Geometry check sheet. Reference: the model listing, model coordinates, mm. Round coordinates to 2 decimals unless told otherwise and drop trailing zeros. Write each loop counter-clockwise with the first axis right and the second up, starting at its lowest first coordinate (ties: lowest second). Pieces come first, ordered by that corner, then holes. Notation, with made-up numbers: (57, 65.25) -> (102, 65.25) arc R22 ccw to (102, 90.25) -> close; hole circle Ø7 at (57.25, -36). An arc over 180 degrees is marked (long way). One line per question, with ' | ' between items.
```python
from build123d import *

# Parameters (mm, degrees)
SKETCH3_R           = 1
BOSS_EXTRUDE2_DEPTH = 1.5
MOVE_FACE1_BY       = 0.2
MOVE_FACE1_2_BY     = 0.2


with BuildPart() as part:
    # Sketch3 → Boss-Extrude2 (new body)
    with BuildSketch(Plane(origin=(0, 0, 0), x_dir=(1, 0, 0), z_dir=(0, 1, 0))):
        with BuildLine():
            Line((9.052045009, -11.69440211), (-2.494704275, -15.782345478))
            Line((-2.494704275, -15.782345478), (-2.714831854, -15.909670913))
            Line((-2.714831854, -15.909670913), (-5.018414472, -17.242101226))
            ThreePointArc((-5.018414472, -17.242101226), (-5.90236336, -19.640824396), (-3.706036939, -20.949024969))
            Line((-3.706036939, -20.949024969), (-1.077229318, -20.535220782))
            Line((-1.077229318, -20.535220782), (-0.82602363, -20.495678153))
            Line((-0.82602363, -20.495678153), (10.720725655, -16.407734785))
            Line((10.720725655, -16.407734785), (13.853836403, -15.298506639))
            ThreePointArc((13.853836403, -15.298506639), (14.422653253, -14.786418923), (14.462766809, -14.022103975))
            Line((14.462766809, -14.022103975), (14.300666867, -13.564238683))
            Line((14.300666867, -13.564238683), (13.487374274, -11.195126647))
            ThreePointArc((13.487374274, -11.195126647), (12.976450881, -10.619337061), (12.207817887, -10.577150797))
            Line((12.207817887, -10.577150797), (9.052045009, -11.69440211))
        make_face()
        with Locations(Location((-4.01703029, -18.973352138, 0), (0, 0, 270))):
            Circle(SKETCH3_R, mode=Mode.SUBTRACT)
        with Locations(Location((12.007385036, -13.300162157, 0), (0, 0, 270))):
            Circle(SKETCH3_R, mode=Mode.SUBTRACT)
    extrude(amount=BOSS_EXTRUDE2_DEPTH)

    # Move Face1: a curved face moved inward by 0.2
    add(Solid.thicken(part.faces().sort_by_distance((12.007385036, 0.75, 12.300162157))[0], -MOVE_FACE1_BY), mode=Mode.SUBTRACT)

    # Move Face1 2: a curved face moved inward by 0.2
    add(Solid.thicken(part.faces().sort_by_distance((-4.01703029, 0.75, 17.973352138))[0], -MOVE_FACE1_2_BY), mode=Mode.SUBTRACT)


solid = part.part
```
(1) Sectioned sample at B-B on z = 13. Record the cut outline in (x, y).
Resolved:
outline: (5.36, 0) -> (10.85, 0) -> (10.85, 1.5) -> (5.36, 1.5) -> close; (13.17, 0) -> (14.11, 0) -> (14.11, 1.5) -> (13.17, 1.5) -> close
(2) Draft check along Z on faces 1 (the flat face through (13.9, 0.7, 12.4)), 2 (the cylindrical face through (-5.915, 0.74, 19.604)), 3 (the cylindrical face through (-3.66, 0.74, 20.12)), 4 (the cylindrical face through (13.197, 0.74, 13.144)). Enter one of: +Z half, -Z half, draft (parallel to the pull), parting line (faces both ways), or undercut.
Resolved:
face 1: -Z half | face 2: parting line | face 3: undercut | face 4: undercut
(3) Sectioned sample at A-A on y = 1.2. Record the cut outline in (x, z).
Resolved:
outline: (-5.02, 17.24) -> (-2.49, 15.78) -> (12.21, 10.58) arc R1 ccw to (13.49, 11.2) -> (14.3, 13.56) -> (14.46, 14.02) arc R1 ccw to (13.85, 15.3) -> (-0.83, 20.5) -> (-3.71, 20.95) arc R2 ccw to start; hole circle Ø2.4 at (-4.02, 18.97); hole circle Ø2.4 at (12.01, 13.3)
(4) Go/stop test with a flat-tipped pin: pin 1 (1.9 mm diameter, centred on x = 12.01, z = 13.3, fed in from +Y). Record where the tip stops, or that it passes through.
Resolved:
pin 1: passes through
(5) Sectioned sample at C-C on x = 11. Record the cut outline in (y, z), then the cut area to 3 significant figures.
Resolved:
outline: (0, 11) -> (1.5, 11) -> (1.5, 12.65) -> (0, 12.65) -> close; (0, 13.95) -> (1.5, 13.95) -> (1.5, 16.31) -> (0, 16.31) -> close | area: 6.00 mm2
(6) Material ranges on line 1 (Z direction, x = -3.5, y = 0.85); line 2 (Z direction, x = 4, y = 1); line 3 (Z direction, x = -3, y = 1.25), recorded low to high.
Resolved:
line 1: z = 16.36 to 17.89, 20.06 to 20.92 | line 2: z = 13.48 to 18.79 | line 3: z = 16.07 to 18.34, 19.61 to 20.84
(7) Sectioned sample at D-D on x = 6. Record the cut outline in (y, z), then the cut area to 3 significant figures.
Resolved:
outline: (0, 12.77) -> (1.5, 12.77) -> (1.5, 18.08) -> (0, 18.08) -> close | area: 7.96 mm2
